Autodesk Inventor part; units mm, degrees
ref_plane "YZ Plane" through (0, 0, 0) normal (1, 0, 0) x (0, 1, 0)
ref_plane "XZ Plane" through (0, 0, 0) normal (0, 1, 0) x (-1, 0, 0)
ref_plane "XY Plane" through (0, 0, 0) normal (0, 0, 1) x (1, 0, 0)
sketch "Sketch2" plane through (0, 0, 0) normal (0, 0, 1) x (1, 0, 0)
  arc A0 (-4.25, 0) -> (4.25, 0) centre (0, 0) ccw
  line L0 (4.25, 0) -> (7.25, 0)
  line L1 (-4.25, 0) -> (-7.25, 0)
  arc A1 (-4.6904, -0.75) -> (4.6904, -0.75) centre (0, 0) ccw
  line L2 (-7.25, 0) -> (-7.25, -0.75)
  line L3 (-7.25, -0.75) -> (-4.6904, -0.75)
  line L4 (7.25, 0) -> (7.25, -0.75)
  line L5 (7.25, -0.75) -> (4.6904, -0.75)
  dimension "d8" = 8.5
  dimension "d9" = 3
  dimension "d10" = 3
  dimension "d11" = 9.5
  dimension "d12" = 0.75
extrude "Extrusion2" add sketch "Sketch2" along normal blind 2
Source: CAD feature listing. Evaluate the final solid. Frame: model axes, mm. A direction names the side the tool comes from. Round coordinates to 2 decimals unless told otherwise and drop trailing zeros. Write each loop counter-clockwise with the first axis right and the second up, starting at its lowest first coordinate (ties: lowest second). Pieces come first, ordered by that corner, then holes. Notation, with made-up numbers: M 65,88.25 L 69,88.25 A27 ccw 69,105.25 Z; hole C 54,23 d10. An arc over 180 degrees is marked long. Answer as a JSON object with one key per item and string values. Group by question number.
(1) Ray query, line 1 (X direction, y = -1.4, z = 0.75); line 2 (Y direction, x = 6, z = 1.8); line 3 (X direction, y = -3.75, z = 1.35). Return the intervals inside material, ascending. Write a range as [from, to].
(2) Section query A-A on z = 0.7. Output: boundary loops of the cut face in (x, y).
(3) Section query B-B on y = -0.55. Output: boundary loops of the cut face in (x, z).
(4) Section query C-C on x = 0. Output: boundary loops of the cut face in (y, z), then the cut area to 4 significant figures.
(5) Section query D-D on y = -2.5. Output: boundary loops of the cut face in (x, z).
(6) First-contact query: pin 1 (1 mm diameter, centred on y = -1.5, z = 2, fed in from +X); pin 2 (0.6 mm diameter, centred on x = 6, z = 1.5, fed in from -Y). Flat tips, straight axial feed; report the tip coordinate or a pass-through.
(7) Reachability of faces 1 (the flat face through (6, -0.75, 1)), 2 (the flat face through (0, -4.5, 2)), 3 (the flat face through (-6, -0.75, 1)) from +Z, -Z, +X, -X, +Y, -Y: full face, straight path, thin tool, end or side. Return the list, or none.
Computed values:
{
 "1": {"line 1": "[-4.54, -4.01], [4.01, 4.54]", "line 2": "[-0.75, 0]", "line 3": "[-2.92, -2], [2, 2.92]"},
 "2": {"outline": "M -7.25,-0.75 L -4.69,-0.75 A4.75 ccw 4.69,-0.75 L 7.25,-0.75 L 7.25,0 L 4.25,0 A4.25 cw -4.25,0 L -7.25,0 Z"},
 "3": {"outline": "M -7.25,0 L -4.21,0 L -4.21,2 L -7.25,2 Z; M 4.21,0 L 7.25,0 L 7.25,2 L 4.21,2 Z"},
 "4": {"outline": "M -4.75,0 L -4.25,0 L -4.25,2 L -4.75,2 Z", "area": "1.000 mm^2"},
 "5": {"outline": "M -4.04,0 L -3.44,0 L -3.44,2 L -4.04,2 Z; M 3.44,0 L 4.04,0 L 4.04,2 L 3.44,2 Z"},
 "6": {"pin 1": "x = 4.64", "pin 2": "y = -0.75"},
 "7": {"face 1": "+Z, -Z, +X, -Y", "face 2": "+Z, +X, -X, +Y, -Y", "face 3": "+Z, -Z, -X, -Y"}
}
